Source: CAD feature listing. Evaluate the final solid. Frame: model axes, mm. Give positions to 0.01 mm unless a question says otherwise; leave off trailing zeros. Write each loop counter-clockwise with the first axis right and the second up, starting at its lowest first coordinate (ties: lowest second). Pieces come first, ordered by that corner, then holes. Notation, with made-up numbers: (-18.5, 41) -> (8.5, 41) arc R4 cw to (8.5, 47) -> close; hole circle Ø9 at (56.5, 49.5). An arc over 180 degrees is marked (long way). Write item = value, one per line.
from build123d import *

# Parameters (mm, degrees)
F0_R     = 1.5
F1_DEPTH = 2.4


with BuildPart() as f1:
    # F0 (on Top) → F1 (new body)
    with BuildSketch(Plane.XY):
        with BuildLine():
            Line((0, 15.125), (-30, 15.125))
            ThreePointArc((-30, 15.125), (-31.4142135624, 14.5392135624), (-32, 13.125))
            Line((-32, 13.125), (-32, -15.125))
            Line((-32, -15.125), (32, -15.125))
            Line((32, -15.125), (32, 13.125))
            ThreePointArc((32, 13.125), (31.4142135624, 14.5392135624), (30, 15.125))
            Line((30, 15.125), (0, 15.125))
        make_face()
        with Locations((-25, 4.825)):
            Circle(F0_R, mode=Mode.SUBTRACT)
        with BuildLine():
            Line((-2, 10.285), (0, 10.285))
            Line((0, 10.285), (2, 10.285))
            ThreePointArc((2, 10.285), (2.7071067812, 9.9921067812), (3, 9.285))
            Line((3, 9.285), (3, 8.5625))
            ThreePointArc((3, 8.5625), (2.7071067812, 7.8553932188), (2, 7.5625))
            Line((2, 7.5625), (0, 7.5625))
            Line((0, 7.5625), (-2.1, 7.5625))
            ThreePointArc((-2.1, 7.5625), (-2.7363961031, 7.8261038969), (-3, 8.4625))
            Line((-3, 8.4625), (-3, 9.285))
            ThreePointArc((-3, 9.285), (-2.7071067812, 9.9921067812), (-2, 10.285))
        make_face(mode=Mode.SUBTRACT)
        with Locations((25, 4.825)):
            Circle(F0_R, mode=Mode.SUBTRACT)
        Polygon((32, -15.125), (-32, -15.125), (-32, -19.125), (-15, -19.125), (0, -19.125), (15, -19.125), (32, -19.125), align=None)
        with BuildLine():
            Line((-15, -19.125), (-32, -19.125))
            Line((-32, -19.125), (-21.0726106353, -32.147755533))
            add(Edge.make_bspline(
                [(-21.0726106353, -32.147755533), (-17.3698433438, -32.3941137596), (-11.5299816466, -32.7826604485), (-9.9449620452, -28.3358600834), (-11.3646535712, -27.4993559227), (-12, -27.125)],
                knots=[0, 0, 0, 0, 0.4890736176, 0.7713480383, 1, 1, 1, 1], degree=3))
            Line((-12, -27.125), (-15, -27.125))
            Line((-15, -27.125), (-15, -19.125))
        make_face()
        with BuildLine():
            Line((21.0726106353, -32.147755533), (32, -19.125))
            Line((32, -19.125), (15, -19.125))
            Line((15, -19.125), (15, -27.125))
            Line((15, -27.125), (12, -27.125))
            add(Edge.make_bspline(
                [(21.0726106353, -32.147755533), (17.3698433438, -32.3941137596), (11.5299816466, -32.7826604485), (9.9449620452, -28.3358600834), (11.3646535712, -27.4993559227), (12, -27.125)],
                knots=[0, 0, 0, 0, 0.4890736176, 0.7713480383, 1, 1, 1, 1], degree=3))
        make_face()
    extrude(amount=F1_DEPTH)


solid = f1.part
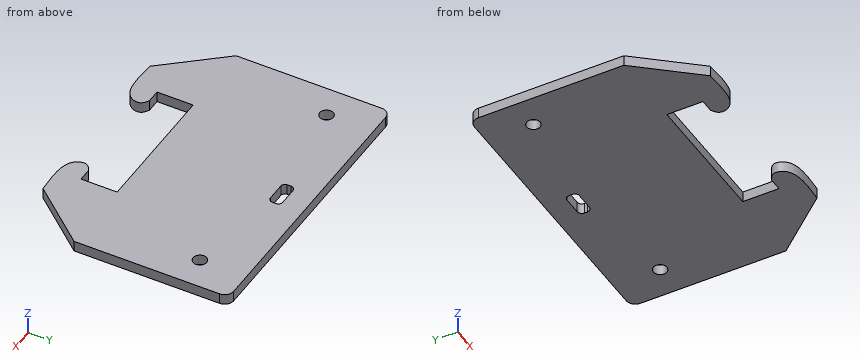
(1) Section query B-B (x = -25). Return loops of the section in (y, z) (3 decimals), plus the area to 3 significant figures.
Values follow:
outline = (-27.467, 0) -> (3.325, 0) -> (3.325, 2.4) -> (-27.467, 2.4) -> close; (6.325, 0) -> (15.125, 0) -> (15.125, 2.4) -> (6.325, 2.4) -> close
area = 95.0 mm2
(2) Section query D-D (x = -7.5). Return loops of the section in (y, z) (3 decimals), plus the area to 3 significant figures.
Values follow:
outline = (-19.125, 0) -> (15.125, 0) -> (15.125, 2.4) -> (-19.125, 2.4) -> close
area = 82.2 mm2
(3) First-contact query: pin 1 (4 mm diameter, centred on x = 25, y = 4.825, fed in from +Z); pin 2 (0.7 mm diameter, centred on x = 0, z = 1.5, fed in from -Y) (3 decimals); pin 3 (0.7 mm diameter, centred on y = -24, z = 1, fed in from +X); pin 4 (1.2 mm diameter, centred on y = -23, z = 1, fed in from -X). Flat tips, straight axial feed; report the tip coordinate or a pass-through.
Values follow:
pin_1 = 2.4
pin_2 = -19.125
pin_3 = 28.2
pin_4 = -29.25
(4) Section query C-C (z = 1.3). Give the number of separate pieces and of enclosed holes in the cut face, plus the area to 3 significant figures.
Values follow:
separate_pieces = 1
enclosed_holes = 3
area = 2,500 mm2
(5) Section query A-A (x = -1). Return loops of the section in (y, z) (1 decimal), plus the area to 3 significant figures.
Values follow:
outline = (-19.1, 0) -> (7.6, 0) -> (7.6, 2.4) -> (-19.1, 2.4) -> close; (10.3, 0) -> (15.1, 0) -> (15.1, 2.4) -> (10.3, 2.4) -> close
area = 75.7 mm2
(6) Material intervals for line 1 (X direction, y = 5, z = 1.8); line 2 (Y direction, x = -5, z = 0.1) (3 decimals); line 3 (X direction, y = -25.5, z = 0.9), sorted ascending.
Values follow:
line_1 = -32 to -26.49, -23.51 to 23.51, 26.49 to 32
line_2 = -19.125 to 15.125
line_3 = -26.65 to -15, 15 to 26.65
